from build123d import *

# Parameters (mm, degrees)
BOSS_EXTRUDE1_DEPTH = 25
SKETCH2_R           = 4
CUT_EXTRUDE1_DEPTH  = 88.229582138
SKETCH3_R           = 1.6
CUT_EXTRUDE2_DEPTH  = 79.755553628
CUT_EXTRUDE3_DEPTH  = 3
FILLET2_R           = 8
CHAMFER2_SIZE       = 10
SKETCH5_W           = 30
SKETCH5_H           = 25
BOSS_EXTRUDE2_DEPTH = 26
SKETCH6_W           = 20.004484435
SKETCH6_H           = 25
BOSS_EXTRUDE3_DEPTH = 40
SKETCH7_W           = 10.4
SKETCH7_H           = 20.4
CUT_EXTRUDE4_DEPTH  = 23
SKETCH9_W           = 20.004484435
SKETCH9_H           = 40
SKETCH9_W_2         = 10.4
SKETCH9_H_2         = 20.4
BOSS_EXTRUDE4_DEPTH = 20
SKETCH10_R          = 2.1
CUT_EXTRUDE6_DEPTH  = 90.566948883
CHAMFER5_SIZE       = 5
SKETCH11_R          = 2
CUT_EXTRUDE7_DEPTH  = 112.736296699
SKETCH12_W          = 20.004484435
SKETCH12_H          = 20
SKETCH12_R          = 2.1
BOSS_EXTRUDE5_DEPTH = 30
SKETCH13_R          = 1.5
CUT_EXTRUDE8_DEPTH  = 103.986592973


with BuildPart() as part:
    # Sketch1 → Boss-Extrude1 (new body)
    with BuildSketch(Plane(origin=(0, 0, 0), x_dir=(1, 0, 0), z_dir=(0, 1, 0))):
        with BuildLine():
            Line((-13.972375691, -8), (-23.972375691, -8))
            Line((-23.972375691, -8), (-23.972375691, -38))
            Line((-23.972375691, -38), (-3.972375691, -38))
            Line((-3.972375691, -38), (-3.972375691, -78))
            Line((-3.972375691, -78), (6.027624309, -78))
            Line((6.027624309, -78), (6.027624309, -38))
            Line((6.027624309, -38), (26.027624309, -38))
            Line((26.027624309, -38), (26.027624309, -8))
            Line((26.027624309, -8), (16.027624309, -8))
            ThreePointArc((16.027624309, -8), (1.027624309, -23), (-13.972375691, -8))
        make_face()
    extrude(amount=BOSS_EXTRUDE1_DEPTH)

    # Sketch2 → Cut-Extrude1 (cut, through all)
    with BuildSketch(Plane.ZY.offset(3.972375691)):
        with Locations((70, 12.5)):
            Circle(SKETCH2_R)
    extrude(amount=-CUT_EXTRUDE1_DEPTH, mode=Mode.SUBTRACT)

    # Sketch3 → Cut-Extrude2 (cut, through all)
    with BuildSketch(Plane(origin=(0, 0, 8), x_dir=(-1, 0, 0), z_dir=(0, 0, -1))):
        with Locations((-21.027624309, 6.5)):
            Circle(SKETCH3_R)
        with Locations((-21.027624309, 18.5)):
            Circle(SKETCH3_R)
        with Locations((18.972375691, 6.5)):
            Circle(SKETCH3_R)
        with Locations((18.972375691, 18.5)):
            Circle(SKETCH3_R)
    extrude(amount=-CUT_EXTRUDE2_DEPTH, mode=Mode.SUBTRACT)

    # Sketch4 → Cut-Extrude3 (cut)
    with BuildSketch(Plane.XY.offset(38)):
        Polygon((24.277624309, 18.5), (22.652624309, 21.314582562), (19.402624309, 21.314582562), (17.777624309, 18.5), (19.402624309, 15.685417438), (22.652624309, 15.685417438), align=None)
        Polygon((24.277624309, 6.5), (22.652624309, 9.314582562), (19.402624309, 9.314582562), (17.777624309, 6.5), (19.402624309, 3.685417438), (22.652624309, 3.685417438), align=None)
        Polygon((-15.722375691, 18.5), (-17.347375691, 21.314582562), (-20.597375691, 21.314582562), (-22.222375691, 18.5), (-20.597375691, 15.685417438), (-17.347375691, 15.685417438), align=None)
        Polygon((-15.722375691, 6.5), (-17.347375691, 9.314582562), (-20.597375691, 9.314582562), (-22.222375691, 6.5), (-20.597375691, 3.685417438), (-17.347375691, 3.685417438), align=None)
    extrude(amount=-CUT_EXTRUDE3_DEPTH, mode=Mode.SUBTRACT)

    # Fillet2
    fillet2_edges = [part.edges().sort_by_distance(p)[0] for p in [
        (1.027624309, 0, 78),
        (1.027624309, 25, 78),
    ]]
    fillet(fillet2_edges, radius=FILLET2_R)

    # Chamfer2
    chamfer2_edges = [part.edges().sort_by_distance(p)[0] for p in [
        (6.027624309, 12.5, 38),
        (-3.972375691, 12.5, 38),
    ]]
    chamfer(chamfer2_edges, length=CHAMFER2_SIZE)

    # Sketch5 → Boss-Extrude2 (add)
    with BuildSketch(Plane.ZY.offset(23.972375691)):
        with Locations((23, 12.5)):
            Rectangle(SKETCH5_W, SKETCH5_H)
    extrude(amount=BOSS_EXTRUDE2_DEPTH)

    # Sketch6 → Boss-Extrude3 (add)
    with BuildSketch(Plane.XY.offset(38)):
        with Locations((-39.970133473, 12.5)):
            Rectangle(SKETCH6_W, SKETCH6_H)
    extrude(amount=BOSS_EXTRUDE3_DEPTH)

    # Sketch7 → Cut-Extrude4 (cut)
    with BuildSketch(Plane.XZ):
        with Locations((-39.970133474, 58)):
            Rectangle(SKETCH7_W, SKETCH7_H)
    extrude(amount=-CUT_EXTRUDE4_DEPTH, mode=Mode.SUBTRACT)

    # Sketch9 → Boss-Extrude4 (add)
    with BuildSketch(Plane.XZ):
        with Locations((-39.970133473, 58)):
            Rectangle(SKETCH9_W, SKETCH9_H)
        with Locations((-39.970133474, 58)):
            Rectangle(SKETCH9_W_2, SKETCH9_H_2, mode=Mode.SUBTRACT)
    extrude(amount=BOSS_EXTRUDE4_DEPTH)

    # Sketch10 → Cut-Extrude6 (cut, through all)
    with BuildSketch(Plane.XY.offset(78)):
        with Locations((-39.970133474, -9.5)):
            Circle(SKETCH10_R)
        with Locations((-39.970133474, 18.5)):
            Circle(SKETCH10_R)
    extrude(amount=-CUT_EXTRUDE6_DEPTH, mode=Mode.SUBTRACT)

    # Chamfer5
    chamfer5_edges = [part.edges().sort_by_distance(p)[0] for p in [
        (-29.967891256, 12.5, 38),
    ]]
    chamfer(chamfer5_edges, length=CHAMFER5_SIZE)

    # Sketch11 → Cut-Extrude7 (cut, through all)
    with BuildSketch(Plane(origin=(26.027624309, 0, 0), x_dir=(0, 0, -1), z_dir=(1, 0, 0))):
        with Locations((-26, 12.5)):
            Circle(SKETCH11_R)
    extrude(amount=-CUT_EXTRUDE7_DEPTH, mode=Mode.SUBTRACT)

    # Sketch12 → Boss-Extrude5 (add)
    with BuildSketch(Plane(origin=(0, 0, 38), x_dir=(-1, 0, 0), z_dir=(0, 0, -1))):
        with Locations((39.970133473, -10)):
            Rectangle(SKETCH12_W, SKETCH12_H)
        with Locations(Location((39.970133474, -9.5, 0), (0, 0, 180))):
            Circle(SKETCH12_R, mode=Mode.SUBTRACT)
    extrude(amount=BOSS_EXTRUDE5_DEPTH)

    # Sketch13 → Cut-Extrude8 (cut, through all)
    with BuildSketch(Plane.XZ.offset(20)):
        with Locations(Location((-33.970133474, 33, 0), (0, 0, 270))):
            Circle(SKETCH13_R)
        with Locations(Location((-45.970133474, 33, 0), (0, 0, 270))):
            Circle(SKETCH13_R)
    extrude(amount=-CUT_EXTRUDE8_DEPTH, mode=Mode.SUBTRACT)


solid = part.part
The listing builds one solid part. Answer for the finished solid, in the listing's coordinates (mm). A direction names the side the tool comes from. Round coordinates to 2 decimals unless told otherwise and drop trailing zeros. Order: outer loops, then holes, each group sorted by start corner. A loop starts at its lowest first (then second) coordinate and runs counter-clockwise, first axis right, second up. Notation, with made-up numbers: (19.25, 15.25) -> (23.25, 15.25) arc R23 ccw to (23.25, 45.25) -> close; hole circle Ø1 at (-28, -28). An arc over 180 degrees is marked (long way). One line per item, written item: value.
Item 1: Find section D-D, the plane y = -9.5. Give the vertices of the cut face in (x, z).
Taken from the geometry:
outline: (-49.97, 8) -> (-42.07, 8) -> (-42.07, 47.8) -> (-45.17, 47.8) -> (-45.17, 68.2) -> (-42.07, 68.2) -> (-42.07, 78) -> (-49.97, 78) -> close; (-37.87, 8) -> (-29.97, 8) -> (-29.97, 78) -> (-37.87, 78) -> (-37.87, 68.2) -> (-34.77, 68.2) -> (-34.77, 47.8) -> (-37.87, 47.8) -> close; hole circle Ø3 at (-45.97, 33); hole circle Ø3 at (-33.97, 33)
Item 2: Find section A-A, the plane z = 26. Give the vertices of the cut face in (x, y), then the cut area to 3 significant figures.
Taken from the geometry:
outline: (-49.97, -20) -> (-29.97, -20) -> (-29.97, 0) -> (26.03, 0) -> (26.03, 10.5) -> (-49.97, 10.5) -> close; (-49.97, 14.5) -> (26.03, 14.5) -> (26.03, 25) -> (-49.97, 25) -> close; hole circle Ø4.2 at (-39.97, -9.5); hole circle Ø4.2 at (-39.97, 18.5); hole circle Ø3.2 at (-18.97, 6.5); hole circle Ø3.2 at (-18.97, 18.5); hole circle Ø3.2 at (21.03, 6.5); hole circle Ø3.2 at (21.03, 18.5)
area: 1,940 mm2
Item 3: Find section C-C, the plane x = -41. Give the vertices of the cut face in (y, z), then the cut area to 3 significant figures.
Taken from the geometry:
outline: (-20, 8) -> (-11.33, 8) -> (-11.33, 47.8) -> (-20, 47.8) -> close; (-20, 68.2) -> (-11.33, 68.2) -> (-11.33, 78) -> (-20, 78) -> close; (-7.67, 8) -> (16.67, 8) -> (16.67, 47.8) -> (-7.67, 47.8) -> close; (-7.67, 68.2) -> (16.67, 68.2) -> (16.67, 78) -> (-7.67, 78) -> close; (20.33, 8) -> (25, 8) -> (25, 78) -> (20.33, 78) -> (20.33, 68.2) -> (23, 68.2) -> (23, 47.8) -> (20.33, 47.8) -> close; hole circle Ø4 at (12.5, 26)
area: 1,900 mm2
Item 4: For faces 3 (the flat face through (-21.42, 17.11, 36.52)), 4 (the flat face through (-45.17, 2, 58)), 5 (the flat face through (-9.04, 12.32, 42.93)), 6 (the cylindrical face through (-41.518, -8.081, 73.169)), determine the directions among +Z, -Z, +X, -X, +Y, -Y from which every point of the face is accessible in a straight line to the end or side of a thin tool.
Taken from the geometry:
face 3: +Z
face 4: -Y
face 5: +Z, +Y, -Y
face 6: +Z, -Z
Item 5: Given P1, Ø13.5, axis at y = 2, z = 55, coming from the +X side; P2, Ø4.5, axis at x = -17.5, y = 6, coming from the +Z side; P3, Ø1, axis at y = -11, z = 65.5, coming from the +X side; P4, Ø5, axis at x = 0, z = 20, coming from the -Y side, each flat-ended and moving along its own axis, determine where each tip first touches the part or whether it passes through.
Taken from the geometry:
P1: stops at x = 6.03
P2: stops at z = 38
P3: stops at x = -29.97
P4: passes through
Item 6: For a pull along X with two mould halves and no side action, classify faces 1 (the flat face through (1, 12, 78)), 2 (the cylindrical face through (1, 12, 23)) as released by +X, released by -X, zero draft, split by the parting line, or undercut.
Taken from the geometry:
face 1: zero draft
face 2: undercut
Item 7: Find section B-B, the plane y = 12.5. State how many separate pieces and enclosed holes the cut face has, then the cut area to 3 significant figures.
Taken from the geometry:
separate pieces: 3
enclosed holes: 3
area: 2,630 mm2
Item 8: Straight lines are drawn through the part: L1, parallel to X at y = 11.5, z = 66; L2, parallel to X at y = 4, z = 33; L3, parallel to Z at x = -42.5, y = -5. For each, find the intervals that lie inside material, in ascending order.
Taken from the geometry:
L1: x = -49.97 to -45.17, -34.77 to -29.97, -3.97 to 6.03
L2: x = -49.97 to -47.47, -44.47 to -35.47, -32.47 to 26.03
L3: z = 8 to 47.8, 68.2 to 78
